Verification items for the finished model (mm, model axes). Face numbers are marked on the shaded views. A direction names the side the tool comes from. Coordinates: 2 decimals unless noted, no trailing zeros. Order: outer loops, then holes, each group sorted by start corner. A loop starts at its lowest first (then second) coordinate and runs counter-clockwise, first axis right, second up. Notation, with made-up numbers: (55, -6) -> (74, -6) arc R38 cw to (74, 32) -> close; hole circle Ø4 at (-33, 4.5). An arc over 180 degrees is marked (long way). Use CSV: the item, a comma, the result in double quotes. Start each with the question number.
1) Tool access check on the marked faces 4 and 5. Record the directions out of +Z, -Z, +X, -X, +Y, -Y that give a thin tool (end or side, any length) a straight path to the whole face; none if there is none.
2) Release check for a two-part mould opening along X. For the marked faces 1, 2 and 3 record: released by +X, released by -X, zero draft, split by the parting line, or undercut.
3) Sectioned sample at D-D on y = -5.75. Record the boundary of the cut face in (x, z), then the cut area to 3 significant figures.
4) Scan lines: line 1 along Y through (x, z) = (8.5, 3.25); line 2 along Y through (x, z) = (-0.5, 1.5); line 3 along Y through (x, z) = (4.5, 3). Record each from-to range of solid material in increasing order.
5) Sectioned sample at A-A on y = 4. Record the boundary of the cut face in (x, z), then the cut area to 3 significant figures.
6) Sectioned sample at C-C on x = 7. Record the boundary of the cut face in (y, z).
7) Go/stop test with flat-tipped pins: pin 1 (6 mm diameter, centred on x = -13.5, z = 4, fed in from -Y); pin 2 (6 mm diameter, centred on x = 6.5, z = 7, fed in from -Y); pin 3 (3 mm diameter, centred on x = -0.5, z = 6, fed in from +Y). Record where each tip stops, or that it passes through.
8) Sectioned sample at B-B on z = 3.5. Record the boundary of the cut face in (x, y), then the cut area to 3 significant figures.
from build123d import *

# Parameters (mm, degrees)
F1_DEPTH = 10
F2_R     = 1


# Not quite as in the source:
# - a feature names something its author has since deleted; it is built from what else it names


with BuildPart() as f1:
    # F0 (on Top) → F1 (new body)
    with BuildSketch(Plane.XY):
        Polygon((2.3, -5), (17.5, -5), (17.5, 5), (2.45, 5), (5.05, 1), (-5.25, 1), (-2.65, 5), (-17.5, 5), (-17.5, -5), (-2.5, -5), align=None)
        Polygon((4.45, -9), (2.3, -5), (-2.5, -5), (-4.65, -9), align=None)
    extrude(amount=F1_DEPTH)

    # F2
    f2_edges = [f1.edges().sort_by_distance(p)[0] for p in [
        (-2.65, 5, 5),
        (2.45, 5, 5),
        (4.45, -9, 5),
        (-4.65, -9, 5),
    ]]
    fillet(f2_edges, radius=F2_R)


solid = f1.part
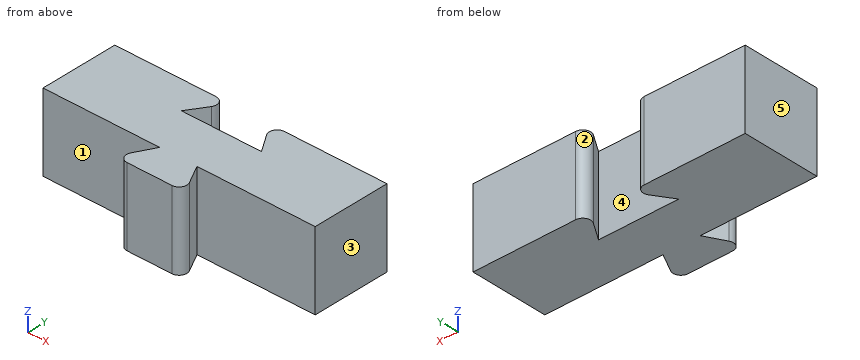
Answers follow:
1,face 4,"+Z, -Z"
1,face 5,"+Z, -Z, -X, +Y, -Y"
2,face 1,"zero draft"
2,face 2,"undercut"
2,face 3,"released by +X"
3,outline,"(-2.9, 0) -> (2.7, 0) -> (2.7, 10) -> (-2.9, 10) -> close"
3,area,"56.1 mm²"
4,line 1,"y = -5 to 5"
4,line 2,"y = -9 to 1"
4,line 3,"y = -5 to 1, 1.85 to 5"
5,outline,"(-17.5, 0) -> (-3.49, 0) -> (-3.49, 10) -> (-17.5, 10) -> close; (3.29, 0) -> (17.5, 0) -> (17.5, 10) -> (3.29, 10) -> close"
5,area,"282 mm²"
6,outline,"(-5, 0) -> (5, 0) -> (5, 10) -> (-5, 10) -> close"
7,pin 1,"stops at y = -5"
7,pin 2,"stops at y = -8.69"
7,pin 3,"stops at y = 1"
8,outline,"(-17.5, -5) -> (-2.5, -5) -> (-3.86, -7.53) arc R1 ccw to (-2.98, -9) -> (2.78, -9) arc R1 ccw to (3.66, -7.53) -> (2.3, -5) -> (17.5, -5) -> (17.5, 5) -> (4.29, 5) arc R1 ccw to (3.45, 3.46) -> (5.05, 1) -> (-5.25, 1) -> (-3.65, 3.46) arc R1 ccw to (-4.49, 5) -> (-17.5, 5) -> close"
8,area,"344 mm²"
